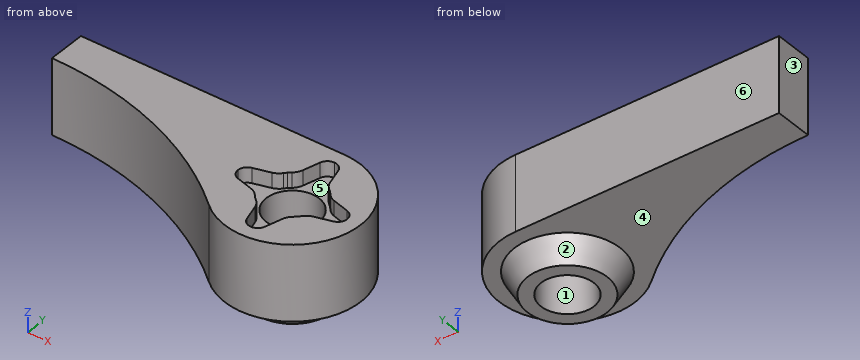
from build123d import *

# Parameters (mm, degrees)
SKETCH1_R             = 9
BOSS_EXTRUDE1_DEPTH   = 10
BODY_MOVE_COPY1_ANGLE = 180
CUT_EXTRUDE5_DEPTH    = 2
SKETCH19_R            = 7
BOSS_EXTRUDE12_DEPTH  = 3
BOSS_EXTRUDE12_TAPER  = 30
SKETCH20_R            = 3.5
CUT_EXTRUDE6_DEPTH    = 39.405728739


with BuildPart() as part:
    # Sketch1 → Boss-Extrude1 (new body)
    with BuildSketch(Plane.XY):
        Circle(SKETCH1_R)
        with BuildLine():
            Line((-35, -9), (0, -9))
            ThreePointArc((0, -9), (-8.437416666, -3.132091953), (-5.872614409, 6.82))
            ThreePointArc((-5.872614409, 6.82), (-19.465199243, -1.204217751), (-35, -4))
            Line((-35, -4), (-35, -9))
        make_face()
    extrude(amount=BOSS_EXTRUDE1_DEPTH)


with BuildPart() as part_1:
    # Body-Move/Copy1: moved
    add(part.part.rotate(Axis((0, 0, 3.5), (1, 0, 0)), BODY_MOVE_COPY1_ANGLE))

    # Sketch18 → Cut-Extrude5 (cut)
    with BuildSketch(Plane.XY.offset(7)):
        with BuildLine():
            Line((1.2, -6.33), (1.8, -4.1378116))
            ThreePointArc((1.8, -4.1378116), (2.058560194, -3.569045514), (2.48, -3.1078116))
            ThreePointArc((2.48, -3.1078116), (2.64989874, -2.964295475), (2.811558399, -2.811558399))
            ThreePointArc((2.811558399, -2.811558399), (2.964295475, -2.64989874), (3.1078116, -2.48))
            ThreePointArc((3.1078116, -2.48), (3.569045514, -2.058560194), (4.1378116, -1.8))
            Line((4.1378116, -1.8), (6.33, -1.2))
            ThreePointArc((6.33, -1.2), (6.992020752, -0.754882576), (7.25, 0))
            ThreePointArc((7.25, 0), (6.992020752, 0.754882576), (6.33, 1.2))
            Line((6.33, 1.2), (4.1378116, 1.8))
            ThreePointArc((4.1378116, 1.8), (3.569045514, 2.058560194), (3.1078116, 2.48))
            ThreePointArc((3.1078116, 2.48), (2.964295475, 2.64989874), (2.811558399, 2.811558399))
            ThreePointArc((2.811558399, 2.811558399), (2.64989874, 2.964295475), (2.48, 3.1078116))
            ThreePointArc((2.48, 3.1078116), (2.058560194, 3.569045514), (1.8, 4.1378116))
            Line((1.8, 4.1378116), (1.2, 6.33))
            ThreePointArc((1.2, 6.33), (0.754882576, 6.992020752), (0, 7.25))
            ThreePointArc((0, 7.25), (-0.754882576, 6.992020752), (-1.2, 6.33))
            Line((-1.2, 6.33), (-1.8, 4.1378116))
            ThreePointArc((-1.8, 4.1378116), (-2.058560194, 3.569045514), (-2.48, 3.1078116))
            ThreePointArc((-2.48, 3.1078116), (-2.64989874, 2.964295475), (-2.811558399, 2.811558399))
            ThreePointArc((-2.811558399, 2.811558399), (-2.964295475, 2.64989874), (-3.1078116, 2.48))
            ThreePointArc((-3.1078116, 2.48), (-3.569045514, 2.058560194), (-4.1378116, 1.8))
            Line((-4.1378116, 1.8), (-6.33, 1.2))
            ThreePointArc((-6.33, 1.2), (-6.992020752, 0.754882576), (-7.25, 0))
            ThreePointArc((-7.25, 0), (-6.992020752, -0.754882576), (-6.33, -1.2))
            Line((-6.33, -1.2), (-4.1378116, -1.8))
            ThreePointArc((-4.1378116, -1.8), (-3.569045514, -2.058560194), (-3.1078116, -2.48))
            ThreePointArc((-3.1078116, -2.48), (-2.964295475, -2.64989874), (-2.811558399, -2.811558399))
            ThreePointArc((-2.811558399, -2.811558399), (-2.64989874, -2.964295475), (-2.48, -3.1078116))
            ThreePointArc((-2.48, -3.1078116), (-2.058560194, -3.569045514), (-1.8, -4.1378116))
            Line((-1.8, -4.1378116), (-1.2, -6.33))
            ThreePointArc((-1.2, -6.33), (-0.754882576, -6.992020752), (0, -7.25))
            ThreePointArc((0, -7.25), (0.754882576, -6.992020752), (1.2, -6.33))
        make_face()
    extrude(amount=-CUT_EXTRUDE5_DEPTH, mode=Mode.SUBTRACT)

    # Sketch19 → Boss-Extrude12 (add)
    with BuildSketch(Plane(origin=(0, 0, -3), x_dir=(-1, 0, 0), z_dir=(0, 0, -1))):
        Circle(SKETCH19_R)
    extrude(amount=BOSS_EXTRUDE12_DEPTH, taper=BOSS_EXTRUDE12_TAPER)

    # Sketch20 → Cut-Extrude6 (cut, through all)
    with BuildSketch(Plane(origin=(0, 0, -6), x_dir=(-1, 0, 0), z_dir=(0, 0, -1))):
        with Locations(Location((0, 0, 0), (0, 0, 90))):
            Circle(SKETCH20_R)
    extrude(amount=-CUT_EXTRUDE6_DEPTH, mode=Mode.SUBTRACT)


solid = part_1.part
Work out the finished part from the listing and answer in its coordinate system (mm). Face numbers are marked on the shaded views. A direction names the side the tool comes from. Give positions to 0.01 mm unless a question says otherwise; leave off trailing zeros. Loops run counter-clockwise (first coordinate to the right, second up) from the corner with the lowest first, then second, coordinate; pieces in that order, holes last. Notation, with made-up numbers: (13, 29.5) - (41, 29.5) arc R13 ccw to (41, 50.5) - close; hole circle Ø2 at (-2, -39.5). An arc over 180 degrees is marked (long way). Answer in a Markdown table with one row per item.
(1) Section C-C (z = -5) is taken. Give the vertices of the cut face in (x, y).
Results list:
| item | result |
|---|---|
| outline | circle Ø11.69 at (0, 0); hole circle Ø7 at (0, 0) |
(2) For a pull along Y with two mould halves and no side action, classify the marked faces 1, 2 and 3 as pulls with the +Y half, pulls with the -Y half, needs draft (parallel to the pull), parting line crosses it, or undercut.
Results list:
| item | result |
|---|---|
| face 1 | undercut |
| face 2 | parting line crosses it |
| face 3 | needs draft |
(3) Flat-ended cylindrical pins translate along their axes: pin 1 Ø6 at (x, z) = (3.5, 3) entering from +Y; pin 2 Ø10 at (x, y) = (-28.5, 2.5) entering from -Z; pin 3 Ø1.5 at (y, z) = (-2, 1) entering from +X. Find the tip coordinate at first contact, or state that the pin passes through.
Results list:
| item | result |
|---|---|
| pin 1 | stops at y = 8.99 |
| pin 2 | stops at z = -3 |
| pin 3 | stops at x = 8.91 |
(4) A tool of negligible diameter and unlimited length cuts with its end or side. For the marked faces 4, 5 and 6, from which of +Z, -Z, +X, -X, +Y, -Y can it reach the whole face along a straight path? Write none if from no direction.
Results list:
| item | result |
|---|---|
| face 4 | -Z |
| face 5 | +Z |
| face 6 | +Z, -Z, +X, -X, +Y |
(5) Section A-A (z = 4.25) is taken. Give the vertices of the cut face in (x, y).
Results list:
| item | result |
|---|---|
| outline | (-35, 4) arc R44.67 cw to (-5.87, -6.82) arc R9 ccw (long way) to (0, 9) - (-35, 9) - close; hole circle Ø7 at (0, 0) |
(6) Consider L1, parallel to Z at x = 4.5, y = -7; L2, parallel to Y at x = 2, z = 2; L3, parallel to X at y = -2, z = -4.25. Determine where each line is inside the solid, lowest interval first. Write a range as [from, to].
Results list:
| item | result |
|---|---|
| L1 | z = [-3, 7] |
| L2 | y = [-8.77, -2.87], [2.87, 8.77] |
| L3 | x = [-5.95, -2.87], [2.87, 5.95] |
(7) Section B-B (x = -14.5) is taken. Give the vertices of the cut face in (y, z).
Results list:
| item | result |
|---|---|
| outline | (-0.99, -3) - (9, -3) - (9, 7) - (-0.99, 7) - close |
